```python
from build123d import *

# Parameters (mm, degrees)
F0_W     = 70
F0_H     = 120
F1_DEPTH = 4
F2_R     = 5
F3_W     = 50
F3_H     = 10.5
F4_DEPTH = 25
F5_R     = 1


with BuildPart() as f1:
    # F0 (on Front) → F1 (new body)
    with BuildSketch(Plane.XZ):
        Rectangle(F0_W, F0_H)
        with BuildLine():
            ThreePointArc((-29, 51.75), (-30.5909902577, 55.5909902577), (-26.75, 54))
            Line((-26.75, 54), (26.75, 54))
            ThreePointArc((26.75, 54), (29, 56.25), (31.25, 54))
            ThreePointArc((31.25, 54), (30.5909902577, 52.4090097423), (29, 51.75))
            Line((29, 51.75), (29, -51.75))
            ThreePointArc((29, -51.75), (30.5909902577, -52.4090097423), (31.25, -54))
            ThreePointArc((31.25, -54), (29, -56.25), (26.75, -54))
            Line((26.75, -54), (-26.75, -54))
            ThreePointArc((-26.75, -54), (-30.5909902577, -55.5909902577), (-29, -51.75))
            Line((-29, -51.75), (-29, 51.75))
        make_face(mode=Mode.SUBTRACT)
        with BuildLine():
            Line((26.75, 54), (-26.75, 54))
            ThreePointArc((-26.75, 54), (-27.4090097423, 52.4090097423), (-29, 51.75))
            Line((-29, 51.75), (-29, -51.75))
            ThreePointArc((-29, -51.75), (-27.4090097423, -52.4090097423), (-26.75, -54))
            Line((-26.75, -54), (26.75, -54))
            ThreePointArc((26.75, -54), (27.4090097423, -52.4090097423), (29, -51.75))
            Line((29, -51.75), (29, 51.75))
            ThreePointArc((29, 51.75), (27.4090097423, 52.4090097423), (26.75, 54))
        make_face()
    extrude(amount=F1_DEPTH)

    # F2
    f2_edges = [f1.edges().sort_by_distance(p)[0] for p in [
        (-35, -2, 60),
        (35, -2, 60),
        (-35, -2, -60),
        (35, -2, -60),
    ]]
    fillet(f2_edges, radius=F2_R)

    # F3 (on face) → F4 (cut)
    with BuildSketch(Plane.XZ.offset(4)):
        with Locations((0, 37.75)):
            Rectangle(F3_W, F3_H)
    extrude(amount=-F4_DEPTH, mode=Mode.SUBTRACT)

    # F5
    f5_edges = [f1.edges().sort_by_distance(p)[0] for p in [
        (-25, -2, 32.5),
        (-25, -2, 43),
        (25, -2, 43),
        (25, -2, 32.5),
    ]]
    fillet(f5_edges, radius=F5_R)


solid = f1.part
```
Check sheet for the modelled part. Datum: model origin and axes. Units: mm. A direction names the side the tool comes from. Round coordinates to 2 decimals unless told otherwise and drop trailing zeros. Order: outer loops, then holes, each group sorted by start corner. A loop starts at its lowest first (then second) coordinate and runs counter-clockwise, first axis right, second up.
1) Tool access check on faces 5 (the flat face through (-25, -2, 38)), 6 (the cylindrical face through (-34, -2, -58)). Record the directions out of +Z, -Z, +X, -X, +Y, -Y that give a thin tool (end or side, any length) a straight path to the whole face; none if there is none.
2) Mould release check, pull along Z, two halves, no side actions. Record for faces 1 (the flat face through (25, -2, 38)), 2 (the flat face through (0, -2, 32.5)), 3 (the flat face through (-35, -2, -1)), 4 (the cylindrical face through (33, -2, -59)): +Z half, -Z half, draft (parallel to the pull), parting line (faces both ways), or undercut.
3) Section check B-B (x = 0.5). Record the boundary of the cut face in (y, z), and give its area (3 significant figures).
4) Section check C-C (y = -2.55). Record the boundary of the cut face in (x, z), and give its area (3 significant figures).
5) Section check A-A (z = 37). Record the boundary of the cut face in (x, y).
6) Scan lines: line 1 (X direction, y = -1.65, z = 54); line 2 (Z direction, x = -29, y = -1.4); line 3 (Z direction, x = -4.5, y = -1.7). Record each from-to range of solid material in increasing order.
Result:
1. face 5: +Y, -Y
1. face 6: -Z, -X, +Y, -Y
2. face 1: undercut
2. face 2: undercut
2. face 3: draft
2. face 4: -Z half
3. outline: (-4, -60) - (0, -60) - (0, 32.5) - (-4, 32.5) - close; (-4, 43) - (0, 43) - (0, 60) - (-4, 60) - close
3. area: 438 mm2
4. outline: (-35, -55) arc R5 ccw to (-30, -60) - (30, -60) arc R5 ccw to (35, -55) - (35, 55) arc R5 ccw to (30, 60) - (-30, 60) arc R5 ccw to (-35, 55) - close; hole circle Ø4.5 at (-29, -54); hole circle Ø4.5 at (-29, 54); hole (-25, 33.5) arc R1 ccw to (-24, 32.5) - (24, 32.5) arc R1 ccw to (25, 33.5) - (25, 42) arc R1 ccw to (24, 43) - (-24, 43) arc R1 ccw to (-25, 42) - close; hole circle Ø4.5 at (29, -54); hole circle Ø4.5 at (29, 54)
4. area: 7,790 mm2
5. outline: (-35, -4) - (-25, -4) - (-25, 0) - (-35, 0) - close; (25, -4) - (35, -4) - (35, 0) - (25, 0) - close
6. line 1: x = -35 to -31.25, -26.75 to 26.75, 31.25 to 35
6. line 2: z = -60 to -56.25, -51.75 to 51.75, 56.25 to 60
6. line 3: z = -60 to 32.5, 43 to 60
